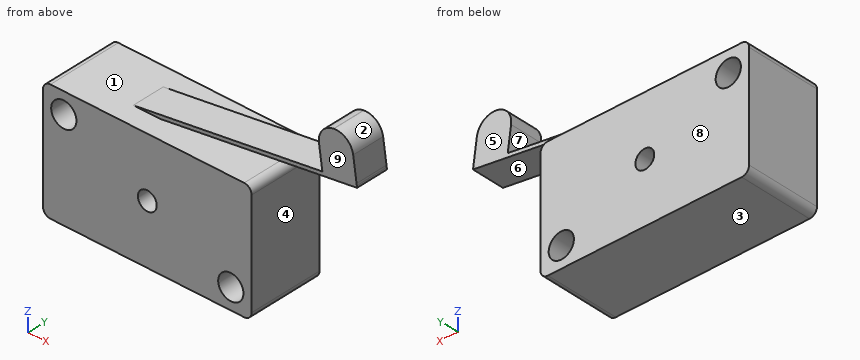
```python
from build123d import *

# Parameters (mm, degrees)
SKETCH1_W               = 28.09
SKETCH1_H               = 16.13
BOSS_EXTRUDE1_DEPTH     = 10.05
BOSS_EXTRUDE2_DEPTH     = 2.215
FILLET1_R               = 1
CUT_EXTRUDE1_DEPTH      = 29.919874566
CUT_EXTRUDE1_DEPTH_BACK = 29.919874566
SKETCH4_R               = 1.7
SKETCH4_R_2             = 1.27
SKETCH6_W               = 4.65
SKETCH6_H               = 4.43
BOSS_EXTRUDE3_DEPTH     = 5.56
FILLET2_R               = 2.3


with BuildPart() as part:
    # Sketch1 → Boss-Extrude1 (new body)
    with BuildSketch(Plane(origin=(0, 0, 0), x_dir=(1, 0, 0), z_dir=(0, 1, 0))):
        Rectangle(SKETCH1_W, SKETCH1_H)
    extrude(amount=BOSS_EXTRUDE1_DEPTH)

    # Sketch3 → Boss-Extrude2 (add, symmetric)
    with BuildSketch(Plane(origin=(0, 5.025, 0), x_dir=(1, 0, 0), z_dir=(0, 1, 0))):
        Polygon((25.656861405, -12.042567225), (25.622068129, -12.290134243), (-4.441324134, -8.065), (-4.371737583, -7.569865966), (25.69165468, -11.795000208), align=None)
    extrude(amount=BOSS_EXTRUDE2_DEPTH, both=True)

    # Fillet1
    fillet1_edges = [part.edges().sort_by_distance(p)[0] for p in [
        (14.045, 5.025, 8.065),
        (-14.045, 5.025, 8.065),
        (-14.045, 5.025, -8.065),
        (14.045, 5.025, -8.065),
    ]]
    fillet(fillet1_edges, radius=FILLET1_R)

    # Sketch4 → Cut-Extrude1 (cut, two sides: drawn at the far end of the back side and taken through both)
    with BuildSketch(Plane(origin=(0, 5.025, 0), x_dir=(1, 0, 0), z_dir=(0, 1, 0)).offset(-CUT_EXTRUDE1_DEPTH_BACK)):
        with Locations(Location((11.245, 5.265, 0), (0, 0, 270))):
            Circle(SKETCH4_R)
        with Locations(Location((-11.245, -5.265, 0), (0, 0, 270))):
            Circle(SKETCH4_R)
        with Locations(Location((0, 0, 0), (0, 0, 270))):
            Circle(SKETCH4_R_2)
    extrude(amount=CUT_EXTRUDE1_DEPTH + CUT_EXTRUDE1_DEPTH_BACK, mode=Mode.SUBTRACT)

    # Sketch6 → Boss-Extrude3 (add)
    with BuildSketch(Plane(origin=(-1.19753232, 0, 8.520885209), x_dir=(0.9902680687415704, 0, 0.13917310096006527), z_dir=(-0.13917310096006527, 0, 0.9902680687415704))):
        with Locations((24.758172017, 5.025)):
            Rectangle(SKETCH6_W, SKETCH6_H)
    extrude(amount=BOSS_EXTRUDE3_DEPTH)

    # Fillet2
    fillet2_edges = [part.edges().sort_by_distance(p)[0] for p in [
        (24.848265688, 5.025, 17.796024705),
        (20.243519168, 5.025, 17.148869785),
    ]]
    fillet(fillet2_edges, radius=FILLET2_R)


solid = part.part
```
Source: CAD feature listing. Evaluate the final solid. Frame: model axes, mm. Face numbers are marked on the shaded views. A direction names the side the tool comes from. Give positions to 0.01 mm unless a question says otherwise; leave off trailing zeros. Order: outer loops, then holes, each group sorted by start corner. A loop starts at its lowest first (then second) coordinate and runs counter-clockwise, first axis right, second up.
(1) Contact query for flat-ended pins moving along their axis: P1, Ø3, axis at y = 5, z = 2.5, coming from the +X side (3 decimals); P2, Ø6, axis at x = 12.5, y = 7.5, coming from the +Z side; P3, Ø5, axis at x = -2.5, y = 3.5, coming from the +Z side. Output: stop coordinate, or through.
(2) Section query D-D (z = -2.75). Return the cut outline in (x, y) (3 decimals), plus the area to 3 significant figures.
(3) Section query C-C (y = 5.25). Return the cut outline in (x, z) (3 decimals).
(4) Material intervals for line 1 along Z through (x, y) = (0, 9) (3 decimals); line 2 along Z through (x, y) = (1, 4.5) (3 decimals); line 3 along X through (y, z) = (6.25, 0) (3 decimals), sorted ascending.
(5) Section query A-A (z = 0). Return the cut outline in (x, y) (3 decimals), plus the area to 3 significant figures.
(6) Section query B-B (x = 2.5). Return the cut outline in (y, z) (3 decimals), plus the area to 3 significant figures.
(7) Access query for the marked faces 5, 6, 7, 8 and 9. Directions: +Z, -Z, +X, -X, +Y, -Y. A direction counts if a zero-diameter tool reaches every point of the face in a straight line with its end or side. Return the directions, or none.
(8) Pull-direction query (Z, two-part tool) for the marked faces 1, 2, 3 and 4; classes: +Z half, -Z half, draft (parallel to the pull), parting line (faces both ways), or undercut.
Outcome:
1. P1: stops at x = 14.045
1. P2: stops at z = 10.87
1. P3: stops at z = 8.69
2. outline: (-14.045, 0) - (14.045, 0) - (14.045, 10.05) - (-14.045, 10.05) - close
2. area: 282 mm2
3. outline: (-14.045, -7.065) arc R1 ccw to (-13.045, -8.065) - (13.045, -8.065) arc R1 ccw to (14.045, -7.065) - (14.045, 7.065) arc R1 ccw to (13.045, 8.065) - (-0.849, 8.065) - (25.692, 11.795) - (25.168, 15.518) arc R2.3 ccw to (22.571, 17.476) - (22.521, 17.469) arc R2.3 ccw to (20.564, 14.871) - (21.017, 11.643) - (-4.441, 8.065) - (-13.045, 8.065) arc R1 ccw to (-14.045, 7.065) - close; hole circle Ø3.4 at (-11.245, 5.265); hole circle Ø2.54 at (0, 0); hole circle Ø3.4 at (11.245, -5.265)
4. line 1: z = -8.065 to -1.27, 1.27 to 8.065
4. line 2: z = -8.065 to -0.783, 0.783 to 8.065, 8.325 to 8.83
4. line 3: x = -14.045 to -1.27, 1.27 to 14.045
5. outline: (-14.045, 0) - (-1.27, 0) - (-1.27, 10.05) - (-14.045, 10.05) - close; (1.27, 0) - (14.045, 0) - (14.045, 10.05) - (1.27, 10.05) - close
5. area: 257 mm2
6. outline: (0, -8.065) - (10.05, -8.065) - (10.05, 8.065) - (0, 8.065) - close; (2.81, 8.536) - (7.24, 8.536) - (7.24, 9.041) - (2.81, 9.041) - close
6. area: 164 mm2
7. face 5: +Z, +X, -X, +Y
7. face 6: +X, +Y, -Y
7. face 7: -X, +Y, -Y
7. face 8: +Z, -Z, +X, -X, +Y
7. face 9: +Z, +X, -X, -Y
8. face 1: undercut
8. face 2: +Z half
8. face 3: -Z half
8. face 4: draft
